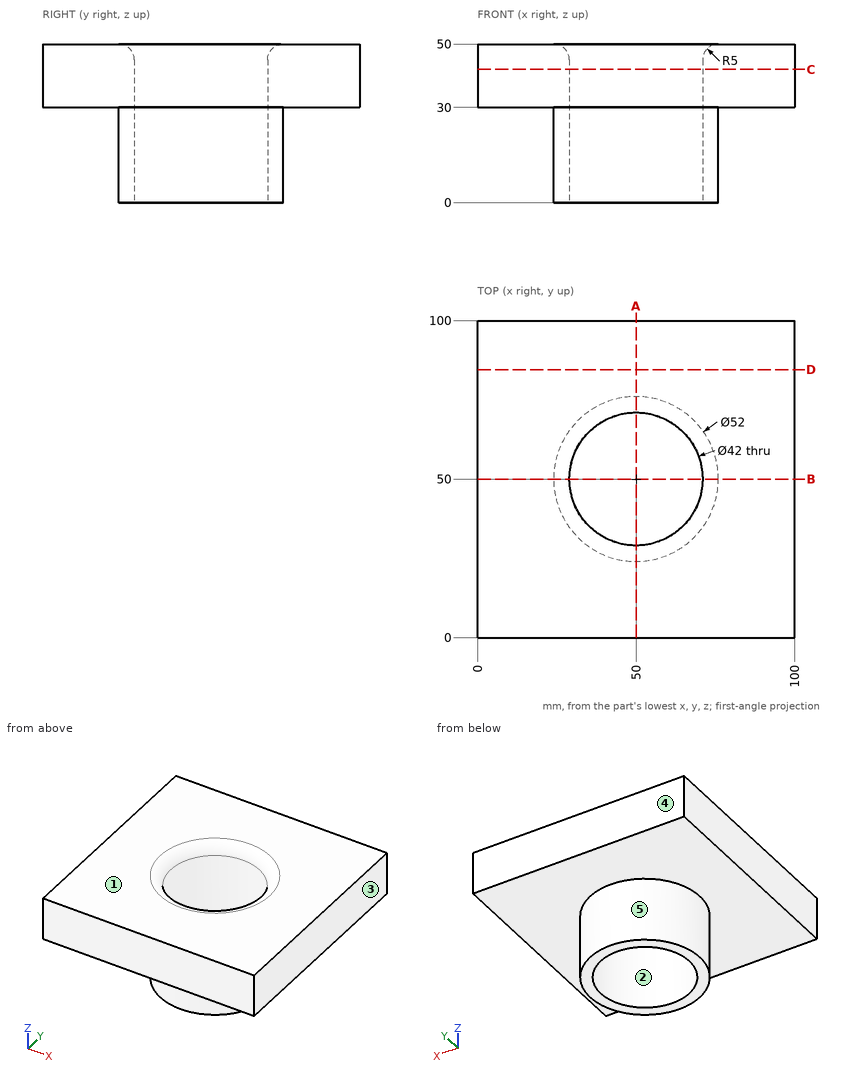
Source: three-view drawing plus pictorial views. Frame: mm from the lowest corner of the part. A direction names the side the tool comes from. Give positions to 0.01 mm unless a question says otherwise; leave off trailing zeros. Order: outer loops, then holes, each group sorted by start corner. A loop starts at its lowest first (then second) coordinate and runs counter-clockwise, first axis right, second up. Notation, with made-up numbers: M 61.5,71.25 L 94.5,71.25 A22 cw 94.5,89.25 Z; hole C 37.5,33 d8. An arc over 180 degrees is marked long. One line per question, with ' | ' between items. Start each with the question number.
1. Pull-direction query (X, two-part tool) for the marked faces 1, 2 and 3; classes: released by +X, released by -X, zero draft, split by the parting line, or undercut.
2. Section query D-D (y = 84.5). Return the cut outline in (x, z).
3. First-contact query: pin 1 Ø6 at (x, z) = (73.5, 33.5) entering from -Y; pin 2 Ø1.5 at (x, z) = (77, 17.5) entering from -Y. Flat tips, straight axial feed; report the tip coordinate or a pass-through.
4. Access query for the marked faces 4 and 5. Directions: +Z, -Z, +X, -X, +Y, -Y. A direction counts if a zero-diameter tool reaches every point of the face in a straight line with its end or side. Return the directions, or none.
5. Section query C-C (z = 42). Return the cut outline in (x, y), and give its area (3 significant figures).
6. Section query A-A (x = 50). Return the cut outline in (y, z).
7. Material intervals for probe 1 along Y at (x, z) = (50, 23); probe 2 along X at (y, z) = (50, 34), sorted ascending. Write a range as [from, to].
Here are the results:
1) face 1: zero draft | face 2: undercut | face 3: released by +X
2) outline: M 0,30 L 100,30 L 100,50 L 0,50 Z
3) pin 1: y = 0 | pin 2: through
4) face 4: +Z, -Z, +X, -X, +Y | face 5: -Z
5) outline: M 0,0 L 100,0 L 100,100 L 0,100 Z; hole C 50,50 d42 | area: 8,610 mm²
6) outline: M 0,30 L 24,30 L 24,0 L 29,0 L 29,45 A5 ccw 24,50 L 0,50 Z; M 71,0 L 76,0 L 76,30 L 100,30 L 100,50 L 76,50 A5 ccw 71,45 Z
7) probe 1: [24, 29], [71, 76] | probe 2: [0, 29], [71, 100]
